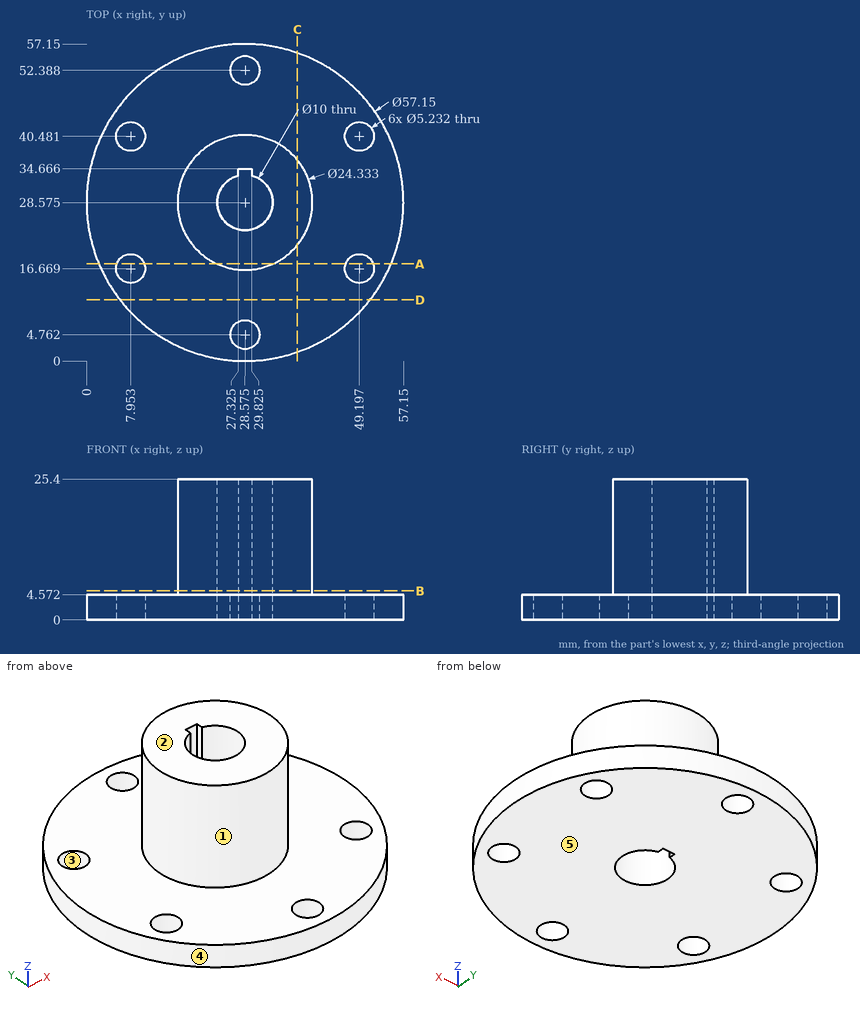
The figure shows three views and two pictorial views of one solid part (mm, origin at its lowest corner). Answer the questions. A direction names the side the tool comes from. Round coordinates to 2 decimals unless told otherwise and drop trailing zeros. Write each loop counter-clockwise with the first axis right and the second up, starting at its lowest first coordinate (ties: lowest second). Pieces come first, ordered by that corner, then holes. Notation, with made-up numbers: (37.5, 4.25) -> (96.5, 4.25) arc R16 ccw to (96.5, 19.25) -> close; hole circle Ø5 at (28.25, 74). An arc over 180 degrees is marked (long way). Answer as a JSON object with one key per item and string values. Group by question number.
Q1. Section B-B (z = 5.25) is taken. Write down the section's boundary in (x, y) (1 decimal).
Q2. Determine the mould class of the marked faces 3, 4 and 5 for opening direction Y: pulls with the +Y half, pulls with the -Y half, needs draft (parallel to the pull), parting line crosses it, or undercut.
Q3. Each of these flat-tipped pins is pushed along its axis until it touches: pin 1 Ø3 at (x, z) = (28, 9) entering from -Y; pin 2 Ø3 at (x, y) = (43, 35) entering from -Z; pin 3 Ø8.5 at (x, y) = (28.58, 4.76) entering from +Z; pin 4 Ø10 at (x, z) = (27, 6) entering from +Y. Where does it stop, or does it pass through?
Q4. Section D-D (y = 11) is taken. Write down the section's boundary in (x, z), plus the area to 3 significant figures.
Q5. Section A-A (y = 17.5) is taken. Write down the section's boundary in (x, z).
Q6. Which of the six approach directions +Z, -Z, +X, -X, +Y, -Y give full straight-line access (tool end or side, diameter ignored) to the marked faces 1 and 2?
Q7. Straight lines are drawn through the part: line 1 along Z through (x, y) = (16.5, 5.5); line 2 along X through (y, z) = (30, 17); line 3 along X through (y, z) = (25, 7.75) (1 decimal). For each, find the intervals that lie inside material, in ascending order.
Q8. Section C-C (x = 38) is taken. Write down the section's boundary in (y, z), plus the area to 3 significant figures.
Check values:
{
 "1": {"outline": "circle Ø24.3 at (28.6, 28.6); hole (27.3, 33.4) arc R5 ccw (long way) to (29.8, 33.4) -> (29.8, 34.7) -> (27.3, 34.7) -> close"},
 "2": {"face 3": "undercut", "face 4": "parting line crosses it", "face 5": "needs draft"},
 "3": {"pin 1": "y = 16.41", "pin 2": "z = 0", "pin 3": "z = 4.57", "pin 4": "y = 57.15"},
 "4": {"outline": "(6.04, 0) -> (51.11, 0) -> (51.11, 4.57) -> (6.04, 4.57) -> close", "area": "206 mm^2"},
 "5": {"outline": "(2.23, 0) -> (5.47, 0) -> (5.47, 4.57) -> (2.23, 4.57) -> close; (10.43, 0) -> (46.72, 0) -> (46.72, 4.57) -> (33.61, 4.57) -> (33.61, 25.4) -> (23.54, 25.4) -> (23.54, 4.57) -> (10.43, 4.57) -> close; (51.68, 0) -> (54.92, 0) -> (54.92, 4.57) -> (51.68, 4.57) -> close"},
 "6": {"face 1": "+Z", "face 2": "+Z, +X, -X, +Y, -Y"},
 "7": {"line 1": "0 to 4.57", "line 2": "16.49 to 23.78, 33.37 to 40.66", "line 3": "16.9 to 25.1, 32.1 to 40.2"},
 "8": {"outline": "(1.6, 0) -> (55.55, 0) -> (55.55, 4.57) -> (36.27, 4.57) -> (36.27, 25.4) -> (20.88, 25.4) -> (20.88, 4.57) -> (1.6, 4.57) -> close", "area": "567 mm^2"}
}
